```python
from build123d import *

# Parameters (mm, degrees)
CROQUIS1_R              = 6.25
CROQUIS1_R_2            = 1.25
SALIENTE_EXTRUIR1_DEPTH = 12.5
CROQUIS2_W              = 7
CROQUIS2_H              = 18.683696708
CORTAR_EXTRUIR1_DEPTH   = 7


with BuildPart() as part:
    # Croquis1 → Saliente-Extruir1 (new body)
    with BuildSketch(Plane.XY):
        with BuildLine():
            Line((41.25, -5.5), (41.25, 5.5))
            ThreePointArc((41.25, 5.5), (8.272659528, 14.321014207), (-15.896844885, 38.428074017))
            Line((-15.896844885, 38.428074017), (-25.423124326, 32.928074017))
            ThreePointArc((-25.423124326, 32.928074017), (-16.573676481, -0.041647684), (-25.36625048, -33.026582408))
            Line((-25.36625048, -33.026582408), (-15.839971039, -38.526582408))
            ThreePointArc((-15.839971039, -38.526582408), (8.287921588, -14.377874913), (41.25, -5.5))
        make_face()
        Circle(CROQUIS1_R, mode=Mode.SUBTRACT)
        with Locations((34.5, 0)):
            Circle(CROQUIS1_R_2, mode=Mode.SUBTRACT)
        with Locations((-17.22811076, -29.930910932)):
            Circle(CROQUIS1_R_2, mode=Mode.SUBTRACT)
        with Locations((-17.284984605, 29.832402542)):
            Circle(CROQUIS1_R_2, mode=Mode.SUBTRACT)
    extrude(amount=SALIENTE_EXTRUIR1_DEPTH)

    # Croquis2 → Cortar-Extruir1 (cut)
    with BuildSketch(Plane.XY.offset(12.5)):
        with Locations((34.5, -0.520271759)):
            Rectangle(CROQUIS2_W, CROQUIS2_H)
        Polygon((-11.360290568, -37.319753641), (-7.860290568, -31.257575815), (-24.040846553, -21.915727461), (-27.540846553, -27.977905287), align=None)
        Polygon((-26.639709432, 28.498177047), (-23.139709432, 22.43599922), (-6.959153447, 31.777847574), (-10.459153447, 37.8400254), align=None)
    extrude(amount=-CORTAR_EXTRUIR1_DEPTH, mode=Mode.SUBTRACT)


solid = part.part
```
Design review of the part built by this model. Coordinates are the model's own, in mm. A direction names the side the tool comes from. Coordinates: 2 decimals unless noted, no trailing zeros. Order: outer loops, then holes, each group sorted by start corner. A loop starts at its lowest first (then second) coordinate and runs counter-clockwise, first axis right, second up.
1) Take a section at C-C, the plane y = 0. Give the boundary of the cut face in (x, z).
2) Take a section at D-D, the plane x = 34.5. Give the boundary of the cut face in (y, z), and give its area (3 significant figures).
3) Take a section at B-B, the plane x = 0. Give the boundary of the cut face in (y, z), and give its area (3 significant figures).
4) Clearance check with flat-ended pins moving along their axes: pin 1 (3 mm diameter, centred on y = 28.5, z = 11, fed in from +X); pin 2 (4 mm diameter, centred on y = -22.5, z = 2, fed in from -X); pin 3 (1.5 mm diameter, centred on x = 5, y = 18, fed in from -Z); pin 4 (4 mm diameter, centred on x = 34.5, y = 0, fed in from +Z). State where each tip first meets the part, or that it passes through.
5) For faces 4 (the flat face through (-19, 30, 5.5)), 5 (the flat face through (-19.03, -32.89, 9.05)), 6 (the flat face through (33.7, -1.3, 5.5)), 7 (the flat face through (-15.615, 26.781, 9.049)), list the 3-axis set-ups (+Z, -Z, +X, -X, +Y, -Y) from which the entire face can be reached by the end or side of a thin tool; tool diameter is ignored.
6) Wall thickness on line 1 along X through (y, z) = (0.5, 11.5); line 2 along Y through (x, z) = (-5.5, 9.25); line 3 along Z through (x, y) = (-20, 31): over which ranges is each line inside the solid? List them lowest first.
7) Take a section at A-A, the plane z = 8. Give the boundary of the cut face in (x, y), and give its area (3 significant figures).
8) Mouldability with a two-part tool opening along Y and no side actions: class faces 1 (the cylindrical face through (7.87, -14.62, 6.16)), 2 (the flat face through (-15.39, -26.91, 9.05)), 3 (the flat face through (38, 0, 9)) as +Y half, -Y half, draft (parallel to the pull), parting line (faces both ways), or undercut.
Returned:
1. outline: (-16.57, 0) - (-6.25, 0) - (-6.25, 12.5) - (-16.57, 12.5) - close; (6.25, 0) - (33.25, 0) - (33.25, 5.5) - (31, 5.5) - (31, 12.5) - (6.25, 12.5) - close; (35.75, 0) - (41.25, 0) - (41.25, 12.5) - (38, 12.5) - (38, 5.5) - (35.75, 5.5) - close
2. outline: (-5.86, 0) - (-1.25, 0) - (-1.25, 5.5) - (-5.86, 5.5) - close; (1.25, 0) - (5.85, 0) - (5.85, 5.5) - (1.25, 5.5) - close
2. area: 50.6 mm2
3. outline: (-20.05, 0) - (-6.25, 0) - (-6.25, 12.5) - (-20.05, 12.5) - close; (6.25, 0) - (19.96, 0) - (19.96, 12.5) - (6.25, 12.5) - close
3. area: 344 mm2
4. pin 1: stops at x = -7.52
4. pin 2: stops at x = -21.25
4. pin 3: passes through
4. pin 4: stops at z = 5.5
5. face 4: +Z
5. face 5: +Z, +X
5. face 6: +Z, +Y, -Y
5. face 7: +Z, -X
6. line 1: x = -16.58 to -6.23, 6.23 to 31, 38 to 41.25
6. line 2: y = -25 to -2.97, 2.97 to 24.89
6. line 3: z = 0 to 5.5
7. outline: (-25.42, 32.93) arc R66.05 cw to (-23.88, 30.09) - (-14.21, 35.67) arc R66.05 cw to (-15.9, 38.43) - close; (-25.37, -33.03) - (-15.84, -38.53) arc R66.05 cw to (-14.13, -35.72) - (-23.8, -30.14) arc R66.05 cw to start; (-21, 23.67) arc R66.05 cw to (-20.94, -23.71) - (-10, -30.02) arc R66.05 cw to (31, -6.32) - (31, 6.3) arc R66.05 cw to (-10.08, 29.98) - close; (38, -5.59) arc R66.05 cw to (41.25, -5.5) - (41.25, 5.5) arc R66.05 cw to (38, 5.58) - close; hole circle Ø12.5 at (0, 0)
7. area: 1,640 mm2
8. face 1: -Y half
8. face 2: undercut
8. face 3: draft
